Geometry check sheet. Reference: the model listing, model coordinates, mm. Face numbers are marked on the shaded views. A direction names the side the tool comes from. Give positions to 0.01 mm unless a question says otherwise; leave off trailing zeros. Order: outer loops, then holes, each group sorted by start corner. A loop starts at its lowest first (then second) coordinate and runs counter-clockwise, first axis right, second up. Notation, with made-up numbers: M 28,83 L 77,83 A20 ccw 77,106 Z; hole C 29.5,51 d10. An arc over 180 degrees is marked long. Put each result on its own line as item: value. Start each with the question number.
Q1. Go/stop test with flat-tipped pins: pin 1 (0.6 mm diameter, centred on x = 5, z = 28, fed in from -Y); pin 2 (4 mm diameter, centred on x = 0.5, z = 24, fed in from +Y); pin 3 (1.5 mm diameter, centred on y = 6.5, z = 13.5, fed in from +X); pin 4 (0.5 mm diameter, centred on y = 4.5, z = 24, fed in from +X). Record where each tip stops, or that it passes through.
Q2. Material ranges on L1, parallel to Z at x = 0.5, y = 5.25; L2, parallel to X at y = 4.5, z = 21; L3, parallel to Z at x = -0.75, y = 1.25, recorded low to high.
Q3. Section check C-C on x = 6.75. Record the cut outline in (y, z).
Q4. Section check D-D on z = 26. Record the cut outline in (x, y), then the cut area to 3 significant figures.
Q5. Section check B-B on y = 3.5. Record the cut outline in (x, z), then the cut area to 3 significant figures.
Q6. Access from +Z, -Z, +X, -X, +Y, -Y to the whole of each face (thin tool, end or side, straight path). Record for the marked faces 1, 2 and 3.
Q7. Section check A-A on z = 12.5. Record the cut outline in (x, y), then the cut area to 3 significant figures.
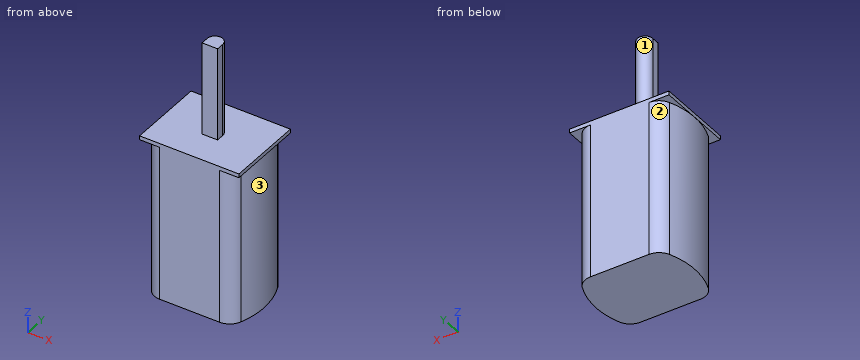
```python
from build123d import *

# Parameters (mm, degrees)
BOSS_EXTRUDE1_DEPTH = 20
BOSS_EXTRUDE2_DEPTH = 0.5
BOSS_EXTRUDE3_DEPTH = 12


with BuildPart() as part:
    # Sketch1 → Boss-Extrude1 (new body)
    with BuildSketch(Plane.XY):
        with BuildLine():
            Line((1.244055551, 0), (8.976470711, 0))
            ThreePointArc((8.976470711, 0), (10.119336086, 0.358702119), (10.85225323, 1.306141266))
            ThreePointArc((10.85225323, 1.306141266), (11.468754399, 5.078261149), (10.62502936, 8.806141266))
            ThreePointArc((10.62502936, 8.806141266), (9.887330043, 9.675154102), (8.794691615, 10))
            Line((8.794691615, 10), (1.244055551, 10))
            ThreePointArc((1.244055551, 10), (0.126021562, 9.658312395), (-0.609994071, 8.75))
            ThreePointArc((-0.609994071, 8.75), (-1.339745962, 5), (-0.609994071, 1.25))
            ThreePointArc((-0.609994071, 1.25), (0.126021562, 0.341687605), (1.244055551, 0))
        make_face()
    extrude(amount=BOSS_EXTRUDE1_DEPTH)

    # Sketch3 → Boss-Extrude2 (add)
    with BuildSketch(Plane.XY.offset(20)):
        Polygon((-1.339745962, 5), (-1.339745962, 0), (11.473340637, 0), (11.473340637, 4.775434937), (11.473340637, 10), (-1.339745962, 10), align=None)
    extrude(amount=BOSS_EXTRUDE2_DEPTH)

    # Sketch4 → Boss-Extrude3 (add)
    with BuildSketch(Plane.XY.offset(20.5)):
        with BuildLine():
            Line((4.065254038, 4), (6.065254038, 4))
            Line((6.065254038, 4), (6.065254038, 5))
            ThreePointArc((6.065254038, 5), (5.065254038, 6), (4.065254038, 5))
            Line((4.065254038, 5), (4.065254038, 4))
        make_face()
    extrude(amount=BOSS_EXTRUDE3_DEPTH)


solid = part.part
```
Results found:
1. pin 1: stops at y = 4
1. pin 2: passes through
1. pin 3: stops at x = 11.43
1. pin 4: stops at x = 6.07
2. L1: z = 0 to 20.5
2. L2: x = 4.07 to 6.07
2. L3: z = 20 to 20.5
3. outline: M 0,0 L 10,0 L 10,20.5 L 0,20.5 Z
4. outline: M 4.07,4 L 6.07,4 L 6.07,5 A1 ccw 4.07,5 Z
4. area: 3.57 mm^2
5. outline: M -1.34,20 L -1.23,20 L -1.23,0 L 11.39,0 L 11.39,20 L 11.47,20 L 11.47,20.5 L -1.34,20.5 Z
5. area: 259 mm^2
6. face 1: +Z, +Y
6. face 2: -Z, -X, +Y
6. face 3: -Z, +X
7. outline: M -0.61,1.25 A2 ccw 1.24,0 L 8.98,0 A2 ccw 10.85,1.31 A10 ccw 10.63,8.81 A2 ccw 8.79,10 L 1.24,10 A2 ccw -0.61,8.75 A10 ccw Z
7. area: 118 mm^2
